```python
from build123d import *

# Parameters (mm, degrees)
SKETCH1_R           = 2
BOSS_EXTRUDE1_DEPTH = 2.4


with BuildPart() as part:
    # Sketch1 → Boss-Extrude1 (new body)
    with BuildSketch(Plane(origin=(0, 0, 0), x_dir=(1, 0, 0), z_dir=(0, 1, 0))):
        with BuildLine():
            Line((-8.5, 14), (8.5, 14))
            ThreePointArc((8.5, 14), (22.5, 0), (8.5, -14))
            Line((8.5, -14), (-8.5, -14))
            ThreePointArc((-8.5, -14), (-22.5, 0), (-8.5, 14))
        make_face()
        with Locations(Location((17.1, 0, 0), (0, 0, 270))):
            Circle(SKETCH1_R, mode=Mode.SUBTRACT)
        with Locations(Location((-17.1, 0, 0), (0, 0, 270))):
            Circle(SKETCH1_R, mode=Mode.SUBTRACT)
    extrude(amount=BOSS_EXTRUDE1_DEPTH)

    # Sketch2 → Revolve1 (revolve)
    with BuildSketch(Plane(origin=(0, 0, 0), x_dir=(0, 0, -1), z_dir=(1, 0, 0)), mode=Mode.PRIVATE) as revolve1_sk:
        with BuildLine():
            Line((-4.621688003, 10.7), (0, 10.7))
            Line((0, 10.7), (0, 2.4))
            Line((0, 2.4), (-9.5, 2.4))
            ThreePointArc((-9.5, 2.4), (-8.190117094, 7.213728491), (-4.621688003, 10.7))
        make_face()
    revolve(revolve1_sk.sketch.rotate(Axis((0, 2.4, 0), (0, 1, 0)), 180), axis=Axis((0, 2.4, 0), (0, 1, 0)))

    # Sketch3 → Revolve2 (revolve)
    with BuildSketch(Plane(origin=(0, 0, 0), x_dir=(0, 0, -1), z_dir=(1, 0, 0))):
        with BuildLine():
            Line((0, 12.8), (0, 2.8))
            ThreePointArc((0, 2.8), (-5, 7.8), (0, 12.8))
        make_face()
    revolve(axis=Axis((0, 12.8, 0), (0, -1, 0)))


solid = part.part
```
Design review of the part built by this model. Coordinates are the model's own, in mm. A direction names the side the tool comes from. Give positions to 0.01 mm unless a question says otherwise; leave off trailing zeros. Write each loop counter-clockwise with the first axis right and the second up, starting at its lowest first coordinate (ties: lowest second). Pieces come first, ordered by that corner, then holes.
(1) Wall thickness on line 1 along X through (y, z) = (0.7, 0); line 2 along Y through (x, z) = (-15, 6.5); line 3 along Z through (x, y) = (-1, 5.75): over which ranges is each line inside the solid? List them lowest first.
Checked values:
line 1: x = -22.5 to -19.1, -15.1 to 15.1, 19.1 to 22.5
line 2: y = 0 to 2.4
line 3: z = -8.83 to 8.83
(2) Add section C-C (z = -7.5). Give the boundary of the cut face in (x, y), and give its area (3 significant figures).
Checked values:
outline: (-20.32, 0) - (20.32, 0) - (20.32, 2.4) - (5.83, 2.4) arc R5.83 ccw to (-5.83, 2.4) - (-20.32, 2.4) - close
area: 151 mm2
(3) Add section D-D (y = 7.75). Give the boundary of the cut face in (x, z).
Checked values:
outline: circle Ø15.7 at (0, 0)
(4) Clearance check with flat-ended pins moving along their axes: pin 1 Ø4 at (x, y) = (1.5, 7) entering from +Z; pin 2 Ø2.5 at (x, z) = (-17.1, 0) entering from +Y; pin 3 Ø2 at (y, z) = (8.5, 1.5) entering from +X; pin 4 Ø4.5 at (x, z) = (17.1, 0) entering from +Y. State where each tip first meets the part, or that it passes through.
Checked values:
pin 1: stops at z = 9.07
pin 2: passes through
pin 3: stops at x = 7.9
pin 4: stops at y = 2.4
(5) Add section B-B (x = 17.1). Give the boundary of the cut face in (y, z), and give its area (3 significant figures).
Checked values:
outline: (0, -11.05) - (2.4, -11.05) - (2.4, -2) - (0, -2) - close; (0, 2) - (2.4, 2) - (2.4, 11.05) - (0, 11.05) - close
area: 43.4 mm2
(6) Tool access review of faces 5 (the face through (15.148, 1.183, -0.434)), 6 (the face through (3, 10.7, -3)): name each direction out of +Z, -Z, +X, -X, +Y, -Y from which nothing blocks a thin tool from reaching the whole face with its end or side.
Checked values:
face 5: +Y, -Y
face 6: +Y
(7) Add section A-A (z = 0). Give the boundary of the cut face in (x, y).
Checked values:
outline: (-22.5, 0) - (-19.1, 0) - (-19.1, 2.4) - (-22.5, 2.4) - close; (-15.1, 0) - (15.1, 0) - (15.1, 2.4) - (9.5, 2.4) arc R9.5 ccw to (4.62, 10.7) - (4.07, 10.7) arc R5 ccw to (-4.07, 10.7) - (-4.62, 10.7) arc R9.5 ccw to (-9.5, 2.4) - (-15.1, 2.4) - close; (19.1, 0) - (22.5, 0) - (22.5, 2.4) - (19.1, 2.4) - close
(8) Mouldability with a two-part tool opening along X and no side actions: class faces 1 (the face through (-22.497, 1.183, 0.308)), 2 (the face through (22.497, 1.183, -0.308)), 3 (the face through (0, 2.4, -10)), 4 (the face through (-15.117, 1.183, -0.26)) as +X half, -X half, draft (parallel to the pull), parting line (faces both ways), or undercut.
Checked values:
face 1: -X half
face 2: +X half
face 3: draft
face 4: undercut
